Geometry: final body of the model. Coordinates: model frame, mm. Face numbers are marked on the shaded views. Give positions to 0.01 mm unless a question says otherwise; leave off trailing zeros. Write each loop counter-clockwise with the first axis right and the second up, starting at its lowest first coordinate (ties: lowest second). Pieces come first, ordered by that corner, then holes.
Q1. Draft query along Y for the marked faces 1 and 2. Return one class per face: pulls with the +Y half, pulls with the -Y half, needs draft (parallel to the pull), parting line crosses it, or undercut.
Q2. Cut plane A-A on x = 0. Return the cut outline in (y, z).
Q3. Pin query (flat end, axial travel): pin 1 (1 mm diameter, centred on x = -24.5, z = 27, fed in from -Y); pin 2 (6 mm diameter, centred on x = 30.05, y = -30.05, fed in from -Z); pin 3 (10.5 mm diameter, centred on x = -30, y = 30.5, fed in from +Z). Return the tip coordinate at first contact, or that it passes through.
Q4. Line query: L1, parallel to X at y = 0.5, z = 13.5; L2, parallel to Y at x = -28, z = 12; L3, parallel to Y at x = 0, z = 0.95. Output: solid intervals per line, ascending.
Q5. Cut plane B-B on z = 35. Return the cut outline in (x, y).
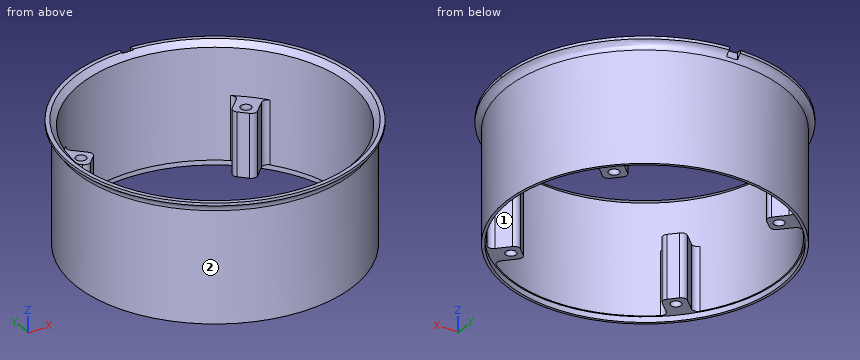
```python
from build123d import *

# Parameters (mm, degrees)
SKETCH2_R                = 50.5
BOSS_EXTRUDE2_DEPTH      = 2
SKETCH3_R                = 50.5
SKETCH3_R_2              = 49
BOSS_EXTRUDE3_DEPTH      = 42
BOSS_EXTRUDE4_START      = -1
SKETCH4_R                = 52.5
SKETCH4_R_2              = 49
BOSS_EXTRUDE4_DEPTH      = 1
FILLET1_R                = 3
CHAMFER1_SIZE            = 2
SKETCH5_R                = 3
SKETCH5_R_2              = 2
SKETCH5_R_3              = 3.125
SKETCH5_R_4              = 3.625
CUT_EXTRUDE3_DEPTH       = 87.304692804
CIRPATTERN1_COUNT        = 4
BOSS_EXTRUDE6_DEPTH      = 25
FILLET3_R                = 2
CIRPATTERN2_COUNT        = 4
FILLET3_OF_CIRPATTERN2_R = 2
CUT_EXTRUDE4_DEPTH       = 87.304692804
SKETCH12_R               = 49.5
CUT_EXTRUDE5_DEPTH       = 2
CUT_EXTRUDE6_REACH       = 88.305
SKETCH10_R               = 1.9
CIRPATTERN3_COUNT        = 4


with BuildPart() as part:
    # Sketch2 → Boss-Extrude2 (new body)
    with BuildSketch(Plane.XY):
        Circle(SKETCH2_R)
    extrude(amount=BOSS_EXTRUDE2_DEPTH)

    # Sketch3 → Boss-Extrude3 (add)
    with BuildSketch(Plane.XY.offset(2)):
        Circle(SKETCH3_R)
        with Locations(Location((0, 0, 0), (0, 0, 180))):
            Circle(SKETCH3_R_2, mode=Mode.SUBTRACT)
    extrude(amount=BOSS_EXTRUDE3_DEPTH)

    # Sketch4 → Boss-Extrude4 (add)
    with BuildSketch(Plane.XY.offset(44).offset(BOSS_EXTRUDE4_START)):
        Circle(SKETCH4_R)
        with Locations(Location((0, 0, 0), (0, 0, 180))):
            Circle(SKETCH4_R_2, mode=Mode.SUBTRACT)
    extrude(amount=BOSS_EXTRUDE4_DEPTH)

    # Fillet1
    # the kernel refuses this fillet: 3 mm, written as the material it adds along each edge
    with BuildSketch(Plane(origin=(0, 0, 43), x_dir=(1, 0, 0), z_dir=(0, 1, 0))) as fillet1_piece_1:
        with BuildLine():
            CenterArc((53.5, 2.828427125), FILLET1_R, 180, 70.528779366)
            Line((52.5, 0), (52.48, -0.056568542))
            ThreePointArc((52.48, -0.056568542), (51.5, -0.06), (50.5, -0.06))
            Line((50.5, -0.06), (50.44, 0))
            Line((50.44, 0), (50.44, 2.828427125))
            Line((50.44, 2.828427125), (50.5, 2.828427125))
        make_face()
    revolve(axis=Axis((0, 0, 43), (0, 0, -1)))

    # Chamfer1
    chamfer1_edges = [part.edges().sort_by_distance(p)[0] for p in [
        (49, 0, 44),
    ]]
    chamfer(chamfer1_edges, length=CHAMFER1_SIZE)

    # Sketch5 → Cut-Extrude3 (cut, through all)
    with BuildSketch(Plane.XY):
        with Locations((0, 20)):
            Circle(SKETCH5_R)
        with Locations((0, 10)):
            Circle(SKETCH5_R_2)
        with Locations((0, 30)):
            Circle(SKETCH5_R_2)
        with Locations((10.125, 20)):
            Circle(SKETCH5_R_3)
        with Locations((-10.125, 20)):
            Circle(SKETCH5_R_4)
    cut_extrude3 = extrude(amount=CUT_EXTRUDE3_DEPTH, mode=Mode.SUBTRACT)

    # CirPattern1: Cut-Extrude3 ×4 about axis
    cirpattern1_axis = Axis((0, 0, 0), (0, 0, 1))
    for i in range(1, CIRPATTERN1_COUNT):
        add(cut_extrude3.rotate(cirpattern1_axis, i * 360 / CIRPATTERN1_COUNT), mode=Mode.SUBTRACT)

    # Sketch7 → Boss-Extrude6 (add)
    with BuildSketch(Plane(origin=(0, 0, 0), x_dir=(-1, 0, 0), z_dir=(0, 0, -1))):
        with BuildLine():
            Line((31.704166175, 37.361020424), (24.748737342, 30.405591591))
            Line((24.748737342, 30.405591591), (30.405591591, 24.748737342))
            Line((30.405591591, 24.748737342), (37.361020424, 31.704166175))
            ThreePointArc((37.361020424, 31.704166175), (34.648232278, 34.648232278), (31.704166175, 37.361020424))
        make_face()
    boss_extrude6 = extrude(amount=-BOSS_EXTRUDE6_DEPTH)

    # Fillet3
    fillet3_edges = [part.edges().sort_by_distance(p)[0] for p in [
        (-30.405591591, 24.748737342, 13.5),
        (-24.748737342, 30.405591591, 13.5),
        (-31.704166175, 37.361020424, 13.5),
        (-37.361020424, 31.704166175, 13.5),
    ]]
    fillet(fillet3_edges, radius=FILLET3_R)

    # CirPattern2: Boss-Extrude6 ×4 about axis
    cirpattern2_axis = Axis((0, 0, 0), (0, 0, 1))
    for i in range(1, CIRPATTERN2_COUNT):
        add(boss_extrude6.rotate(cirpattern2_axis, i * 360 / CIRPATTERN2_COUNT))

    # Fillet3 of CirPattern2
    fillet3_of_cirpattern2_edges = [part.edges().sort_by_distance(p)[0] for p in [
        (-24.748737342, -30.405591591, 13.5),
        (-30.405591591, -24.748737342, 13.5),
        (-37.361020424, -31.704166175, 13.5),
        (-31.704166175, -37.361020424, 13.5),
        (30.405591591, -24.748737342, 13.5),
        (24.748737342, -30.405591591, 13.5),
        (31.704166175, -37.361020424, 13.5),
        (37.361020424, -31.704166175, 13.5),
        (24.748737342, 30.405591591, 13.5),
        (30.405591591, 24.748737342, 13.5),
        (37.361020424, 31.704166175, 13.5),
        (31.704166175, 37.361020424, 13.5),
    ]]
    fillet(fillet3_of_cirpattern2_edges, radius=FILLET3_OF_CIRPATTERN2_R)

    # Sketch9 → Cut-Extrude4 (cut, through all)
    with BuildSketch(Plane.XY):
        with BuildLine():
            Line((-2, 52.46189093), (-2, 50.75))
            Line((-2, 50.75), (2, 50.75))
            Line((2, 50.75), (2, 52.46189093))
            ThreePointArc((2, 52.46189093), (0, 52.5), (-2, 52.46189093))
        make_face()
    extrude(amount=CUT_EXTRUDE4_DEPTH, mode=Mode.SUBTRACT)

    # Sketch12 → Cut-Extrude5 (cut)
    with BuildSketch(Plane.XY):
        Circle(SKETCH12_R)
    extrude(amount=CUT_EXTRUDE5_DEPTH, mode=Mode.SUBTRACT)

    # Sketch10 → Cut-Extrude6 (cut, up to next)
    with BuildSketch(Plane.XY, mode=Mode.PRIVATE) as cut_extrude6_sk1:
        with Locations(Location((-30.0520382, 30.0520382, 0), (0, 0, 180))):
            Circle(SKETCH10_R)
    cut_extrude6_tool1 = extrude(cut_extrude6_sk1.sketch, amount=CUT_EXTRUDE6_REACH, mode=Mode.PRIVATE) & part.part
    cut_extrude6 = cut_extrude6_tool1.solids().sort_by_distance((-30.052038, 30.052038, 0))[0]
    add(cut_extrude6, mode=Mode.SUBTRACT)

    # CirPattern3: Cut-Extrude6 ×4 about axis
    cirpattern3_axis = Axis((0, 0, 0), (0, 0, 1))
    for i in range(1, CIRPATTERN3_COUNT):
        add(cut_extrude6.rotate(cirpattern3_axis, i * 360 / CIRPATTERN3_COUNT), mode=Mode.SUBTRACT)


solid = part.part
```
Data:
1. face 1: undercut
1. face 2: parting line crosses it
2. outline: (-52.5, 43) arc R3 cw to (-50.5, 40.17) - (-50.5, 0) - (-49.5, 0) - (-49.5, 2) - (-49, 2) - (-49, 42) - (-51, 44) - (-52.5, 44) - close; (49, 2) - (49.5, 2) - (49.5, 0) - (50.5, 0) - (50.5, 40.17) arc R3 cw to (50.75, 41.37) - (50.75, 43.75) - (49, 42) - close
3. pin 1: stops at y = -44.43
3. pin 2: stops at z = 2
3. pin 3: stops at z = 25
4. L1: x = -50.5 to -49, 49 to 50.5
4. L2: y = -42.03 to -40.21, -33.66 to -27.15, 27.15 to 33.66, 40.21 to 42.03
4. L3: y = -50.5 to -49.5, 49.5 to 50.5
5. outline: circle Ø101 at (0, 0); hole circle Ø98 at (0, 0)
